from build123d import *

# Parameters (mm, degrees)
SKETCH_1_R      = 10
SKETCH_1_R_2    = 2
EXTRUDE_1_DEPTH = 2


with BuildPart() as part:
    # 草图1 → 凸台-拉伸1 (new body)
    with BuildSketch(Plane.XY):
        Polygon((317.453360513, 257.462931603), (317.453360513, 258.962931603), (314.853360513, 258.962931603), (314.853360513, 257.462931603), (311.853360513, 257.462931603), (311.853360513, 254.462931603), (314.853360513, 254.462931603), (314.853360513, 252.962931603), (317.453360513, 252.962931603), (317.453360513, 254.462931603), (319.953360513, 254.462931603), (319.953360513, 239.462931603), (321.953360513, 239.462931603), (321.953360513, 234.462931603), (319.953360513, 234.462931603), (319.953360513, 229.462931603), (321.953360513, 229.462931603), (321.953360513, 224.462931603), (319.953360513, 224.462931603), (319.953360513, 205.962931603), (301.453360513, 205.962931603), (301.453360513, 203.962931603), (296.453360513, 203.962931603), (296.453360513, 205.962931603), (291.453360513, 205.962931603), (291.453360513, 203.962931603), (286.453360513, 203.962931603), (286.453360513, 205.962931603), (271.453360513, 205.962931603), (271.453360513, 208.462931603), (272.953360513, 208.462931603), (272.953360513, 211.062931603), (271.453360513, 211.062931603), (271.453360513, 214.062931603), (268.453360513, 214.062931603), (268.453360513, 211.062931603), (266.953360513, 211.062931603), (266.953360513, 208.462931603), (268.453360513, 208.462931603), (268.453360513, 205.962931603), (231.453360513, 205.962931603), (231.453360513, 208.462931603), (232.953360513, 208.462931603), (232.953360513, 211.062931603), (231.453360513, 211.062931603), (231.453360513, 214.062931603), (228.453360513, 214.062931603), (228.453360513, 211.062931603), (226.953360513, 211.062931603), (226.953360513, 208.462931603), (228.453360513, 208.462931603), (228.453360513, 205.962931603), (213.453360513, 205.962931603), (213.453360513, 203.962931603), (208.453360513, 203.962931603), (208.453360513, 205.962931603), (203.453360513, 205.962931603), (203.453360513, 203.962931603), (198.453360513, 203.962931603), (198.453360513, 205.962931603), (179.953360513, 205.962931603), (179.953360513, 224.462931603), (177.953360513, 224.462931603), (177.953360513, 229.462931603), (179.953360513, 229.462931603), (179.953360513, 234.462931603), (177.953360513, 234.462931603), (177.953360513, 239.462931603), (179.953360513, 239.462931603), (179.953360513, 254.462931603), (182.453360513, 254.462931603), (182.453360513, 252.962931603), (185.053360513, 252.962931603), (185.053360513, 254.462931603), (188.053360513, 254.462931603), (188.053360513, 257.462931603), (185.053360513, 257.462931603), (185.053360513, 258.962931603), (182.453360513, 258.962931603), (182.453360513, 257.462931603), (179.953360513, 257.462931603), (179.953360513, 294.462931603), (182.453360513, 294.462931603), (182.453360513, 292.962931603), (185.053360513, 292.962931603), (185.053360513, 294.462931603), (188.053360513, 294.462931603), (188.053360513, 297.462931603), (185.053360513, 297.462931603), (185.053360513, 298.962931603), (182.453360513, 298.962931603), (182.453360513, 297.462931603), (179.953360513, 297.462931603), (179.953360513, 312.462931603), (177.953360513, 312.462931603), (177.953360513, 317.462931603), (179.953360513, 317.462931603), (179.953360513, 322.462931603), (177.953360513, 322.462931603), (177.953360513, 327.462931603), (179.953360513, 327.462931603), (179.953360513, 345.962931603), (198.453360513, 345.962931603), (198.453360513, 347.962931603), (203.453360513, 347.962931603), (203.453360513, 345.962931603), (208.453360513, 345.962931603), (208.453360513, 347.962931603), (213.453360513, 347.962931603), (213.453360513, 345.962931603), (228.453360513, 345.962931603), (228.453360513, 343.462931603), (226.953360513, 343.462931603), (226.953360513, 340.862931603), (228.453360513, 340.862931603), (228.453360513, 337.862931603), (231.453360513, 337.862931603), (231.453360513, 340.862931603), (232.953360513, 340.862931603), (232.953360513, 343.462931603), (231.453360513, 343.462931603), (231.453360513, 345.962931603), (268.453360513, 345.962931603), (268.453360513, 343.462931603), (266.953360513, 343.462931603), (266.953360513, 340.862931603), (268.453360513, 340.862931603), (268.453360513, 337.862931603), (271.453360513, 337.862931603), (271.453360513, 340.862931603), (272.953360513, 340.862931603), (272.953360513, 343.462931603), (271.453360513, 343.462931603), (271.453360513, 345.962931603), (286.453360513, 345.962931603), (286.453360513, 347.962931603), (291.453360513, 347.962931603), (291.453360513, 345.962931603), (296.453360513, 345.962931603), (296.453360513, 347.962931603), (301.453360513, 347.962931603), (301.453360513, 345.962931603), (319.953360513, 345.962931603), (319.953360513, 327.462931603), (321.953360513, 327.462931603), (321.953360513, 322.462931603), (319.953360513, 322.462931603), (319.953360513, 317.462931603), (321.953360513, 317.462931603), (321.953360513, 312.462931603), (319.953360513, 312.462931603), (319.953360513, 297.462931603), (317.453360513, 297.462931603), (317.453360513, 298.962931603), (314.853360513, 298.962931603), (314.853360513, 297.462931603), (311.853360513, 297.462931603), (311.853360513, 294.462931603), (314.853360513, 294.462931603), (314.853360513, 292.962931603), (317.453360513, 292.962931603), (317.453360513, 294.462931603), (319.953360513, 294.462931603), (319.953360513, 257.462931603), align=None)
        with Locations((249.953360513, 275.962931603)):
            Circle(SKETCH_1_R, mode=Mode.SUBTRACT)
        with Locations((230.953360513, 275.962931603)):
            Circle(SKETCH_1_R_2, mode=Mode.SUBTRACT)
        with Locations((236.518331671, 289.397960445)):
            Circle(SKETCH_1_R_2, mode=Mode.SUBTRACT)
        with Locations((249.953360513, 294.962931603)):
            Circle(SKETCH_1_R_2, mode=Mode.SUBTRACT)
        with Locations((263.388389356, 289.397960445)):
            Circle(SKETCH_1_R_2, mode=Mode.SUBTRACT)
        with Locations((268.953360513, 275.962931603)):
            Circle(SKETCH_1_R_2, mode=Mode.SUBTRACT)
        with Locations((263.388389356, 262.52790276)):
            Circle(SKETCH_1_R_2, mode=Mode.SUBTRACT)
        with Locations((249.953360513, 256.962931603)):
            Circle(SKETCH_1_R_2, mode=Mode.SUBTRACT)
        with Locations((236.518331671, 262.52790276)):
            Circle(SKETCH_1_R_2, mode=Mode.SUBTRACT)
    extrude(amount=EXTRUDE_1_DEPTH)


solid = part.part
Input: part model. Units: mm. Frame: model coordinates. Give positions to 0.01 mm unless a question says otherwise; leave off trailing zeros. Order: outer loops, then holes, each group sorted by start corner. A loop starts at its lowest first (then second) coordinate and runs counter-clockwise, first axis right, second up. Notation, with made-up numbers: (-37.75, 73) -> (-21.75, 73) arc R32 ccw to (-21.75, 108) -> close; hole circle Ø6 at (57, 18). An arc over 180 degrees is marked (long way). Use one line per item in the form item = value.
1) Line query: probe 1 along Y at (x, z) = (187.5, 1.5); probe 2 along Y at (x, z) = (184.5, 0.95); probe 3 along X at (y, z) = (263, 1.15). Output: solid intervals per line, ascending.
Response values:
probe_1 = 205.96 to 254.46, 257.46 to 294.46, 297.46 to 345.96
probe_2 = 205.96 to 252.96, 258.96 to 292.96, 298.96 to 345.96
probe_3 = 179.95 to 234.57, 238.46 to 261.44, 265.33 to 319.95
2) First-contact query: pin 1 Ø1 at (y, z) = (296.5, 1) entering from -X; pin 2 Ø0.6 at (x, z) = (321, 1) entering from +Y; pin 3 Ø5 at (x, y) = (245.5, 281) entering from -Z; pin 4 Ø1 at (y, z) = (344.5, 0.5) entering from +X. Flat tips, straight axial feed; report the tip coordinate or a pass-through.
Response values:
pin_1 = 188.05
pin_2 = 327.46
pin_3 = through
pin_4 = 319.95
3) Section B-B, the plane y = 331.5. Return loops of the section in (x, z).
Response values:
outline = (179.95, 0) -> (319.95, 0) -> (319.95, 2) -> (179.95, 2) -> close
4) Section C-C, the plane z = 1.4. Count the separate pieces of the cut face and the enclosed holes in it, and give its area (3 significant figures).
Response values:
separate_pieces = 1
enclosed_holes = 9
area = 19,100 mm^2
5) Mould query, pull axis X, two halves, no side actions, for faces 1 (the flat face through (251, 261, 2)), 2 (the cylindrical face through (234.52, 289.49, 0.99)), 3 (the cylindrical face through (259.49, 278.97, 0.99)). Classes: pulls with the +X half, pulls with the -X half, needs draft (parallel to the pull), parting line crosses it, or undercut.
Response values:
face_1 = needs draft
face_2 = undercut
face_3 = undercut
6) Section A-A, the plane x = 283. Return loops of the section in (y, z).
Response values:
outline = (205.96, 0) -> (345.96, 0) -> (345.96, 2) -> (205.96, 2) -> close
